The model under review builds one solid part; all positions refer to its coordinate system, in mm. Round coordinates to 2 decimals unless told otherwise and drop trailing zeros. Order: outer loops, then holes, each group sorted by start corner. A loop starts at its lowest first (then second) coordinate and runs counter-clockwise, first axis right, second up.
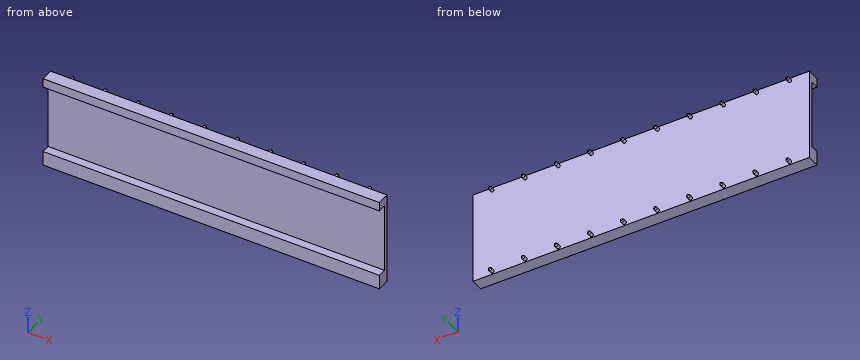
from build123d import *
from OCP.BRepFilletAPI import BRepFilletAPI_MakeChamfer

# Parameters (mm, degrees)
SKETCH1_W                   = 488.315
SKETCH1_H                   = 133.985
BOSS_EXTRUDE1_DEPTH         = 6.0452
SKETCH2_R                   = 2.4765
BOSS_EXTRUDE2_DEPTH         = 7.62
CHAMFER1_SIZE               = 2.032
CHAMFER1_SIZE2              = 1.173175747
LPATTERN1_COUNT             = 5
LPATTERN1_PITCH             = 95.9866
CHAMFER1_OF_LPATTERN1_SIZE  = 2.032
CHAMFER1_OF_LPATTERN1_SIZE2 = 1.173175747
SKETCH3_W                   = 20.955
SKETCH3_H                   = 12.065
SKETCH3_W_2                 = 13.0048
BOSS_EXTRUDE3_DEPTH         = 488.315


with BuildPart() as part:
    # Sketch1 → Boss-Extrude1 (new body)
    with BuildSketch(Plane(origin=(0, 0, 0), x_dir=(1, 0, 0), z_dir=(0, 1, 0))):
        with Locations((244.1575, -66.9925)):
            Rectangle(SKETCH1_W, SKETCH1_H)
    extrude(amount=-BOSS_EXTRUDE1_DEPTH)

    # Sketch2 → Boss-Extrude2 (add)
    with BuildSketch(Plane(origin=(0, 0, 0), x_dir=(1, 0, 0), z_dir=(0, 1, 0))):
        with Locations(Location((28.1305, -4.0005, 0), (0, 0, 90))):
            Circle(SKETCH2_R)
        with Locations(Location((76.1365, -4.0005, 0), (0, 0, 90))):
            Circle(SKETCH2_R)
        with Locations(Location((28.1305, -129.9845, 0), (0, 0, 90))):
            Circle(SKETCH2_R)
        with Locations(Location((76.1365, -129.9845, 0), (0, 0, 90))):
            Circle(SKETCH2_R)
    boss_extrude2 = extrude(amount=BOSS_EXTRUDE2_DEPTH)

    # Chamfer1: one chamfer whose edges measure the first distance from different faces: ONE call of the kernel's chamfer builder (chamfer() names one face for all edges)
    chamfer1_edges_1 = [part.edges().sort_by_distance(p)[0] for p in [
        (28.1305, 7.62, 6.477),
    ]]
    chamfer1_side_1 = [part.faces().sort_by_distance(p)[0] for p in [
        (28.1305, 3.81, 6.477),
    ]]
    chamfer1_edges_2 = [part.edges().sort_by_distance(p)[0] for p in [
        (76.1365, 7.62, 6.477),
    ]]
    chamfer1_side_2 = [part.faces().sort_by_distance(p)[0] for p in [
        (76.1365, 3.81, 6.477),
    ]]
    chamfer1_edges_3 = [part.edges().sort_by_distance(p)[0] for p in [
        (28.1305, 7.62, 132.461),
    ]]
    chamfer1_side_3 = [part.faces().sort_by_distance(p)[0] for p in [
        (28.1305, 3.81, 132.461),
    ]]
    chamfer1_edges_4 = [part.edges().sort_by_distance(p)[0] for p in [
        (76.1365, 7.62, 132.461),
    ]]
    chamfer1_side_4 = [part.faces().sort_by_distance(p)[0] for p in [
        (76.1365, 3.81, 132.461),
    ]]
    chamfer1 = BRepFilletAPI_MakeChamfer(part.part.solid().wrapped)
    for e in chamfer1_edges_1:
        chamfer1.Add(CHAMFER1_SIZE, CHAMFER1_SIZE2, e.wrapped, chamfer1_side_1[0].wrapped)  # the first distance lies on this face
    for e in chamfer1_edges_2:
        chamfer1.Add(CHAMFER1_SIZE, CHAMFER1_SIZE2, e.wrapped, chamfer1_side_2[0].wrapped)  # the first distance lies on this face
    for e in chamfer1_edges_3:
        chamfer1.Add(CHAMFER1_SIZE, CHAMFER1_SIZE2, e.wrapped, chamfer1_side_3[0].wrapped)  # the first distance lies on this face
    for e in chamfer1_edges_4:
        chamfer1.Add(CHAMFER1_SIZE, CHAMFER1_SIZE2, e.wrapped, chamfer1_side_4[0].wrapped)  # the first distance lies on this face
    add(Compound.cast(chamfer1.Shape()), mode=Mode.REPLACE)

    # LPattern1: Boss-Extrude2 ×5
    with Locations(*[(i * LPATTERN1_PITCH, 0, 0) for i in range(1, LPATTERN1_COUNT)]):
        add(boss_extrude2)

    # Chamfer1 of LPattern1: one chamfer whose edges measure the first distance from different faces: ONE call of the kernel's chamfer builder (chamfer() names one face for all edges)
    chamfer1_of_lpattern1_edges_1 = [part.edges().sort_by_distance(p)[0] for p in [
        (124.1171, 7.62, 6.477),
    ]]
    chamfer1_of_lpattern1_side_1 = [part.faces().sort_by_distance(p)[0] for p in [
        (124.1171, 3.81, 6.477),
    ]]
    chamfer1_of_lpattern1_edges_2 = [part.edges().sort_by_distance(p)[0] for p in [
        (172.1231, 7.62, 6.477),
    ]]
    chamfer1_of_lpattern1_side_2 = [part.faces().sort_by_distance(p)[0] for p in [
        (172.1231, 3.81, 6.477),
    ]]
    chamfer1_of_lpattern1_edges_3 = [part.edges().sort_by_distance(p)[0] for p in [
        (124.1171, 7.62, 132.461),
    ]]
    chamfer1_of_lpattern1_side_3 = [part.faces().sort_by_distance(p)[0] for p in [
        (124.1171, 3.81, 132.461),
    ]]
    chamfer1_of_lpattern1_edges_4 = [part.edges().sort_by_distance(p)[0] for p in [
        (172.1231, 7.62, 132.461),
    ]]
    chamfer1_of_lpattern1_side_4 = [part.faces().sort_by_distance(p)[0] for p in [
        (172.1231, 3.81, 132.461),
    ]]
    chamfer1_of_lpattern1_edges_5 = [part.edges().sort_by_distance(p)[0] for p in [
        (220.1037, 7.62, 6.477),
    ]]
    chamfer1_of_lpattern1_side_5 = [part.faces().sort_by_distance(p)[0] for p in [
        (220.1037, 3.81, 6.477),
    ]]
    chamfer1_of_lpattern1_edges_6 = [part.edges().sort_by_distance(p)[0] for p in [
        (268.1097, 7.62, 6.477),
    ]]
    chamfer1_of_lpattern1_side_6 = [part.faces().sort_by_distance(p)[0] for p in [
        (268.1097, 3.81, 6.477),
    ]]
    chamfer1_of_lpattern1_edges_7 = [part.edges().sort_by_distance(p)[0] for p in [
        (220.1037, 7.62, 132.461),
    ]]
    chamfer1_of_lpattern1_side_7 = [part.faces().sort_by_distance(p)[0] for p in [
        (220.1037, 3.81, 132.461),
    ]]
    chamfer1_of_lpattern1_edges_8 = [part.edges().sort_by_distance(p)[0] for p in [
        (268.1097, 7.62, 132.461),
    ]]
    chamfer1_of_lpattern1_side_8 = [part.faces().sort_by_distance(p)[0] for p in [
        (268.1097, 3.81, 132.461),
    ]]
    chamfer1_of_lpattern1_edges_9 = [part.edges().sort_by_distance(p)[0] for p in [
        (316.0903, 7.62, 6.477),
    ]]
    chamfer1_of_lpattern1_side_9 = [part.faces().sort_by_distance(p)[0] for p in [
        (316.0903, 3.81, 6.477),
    ]]
    chamfer1_of_lpattern1_edges_10 = [part.edges().sort_by_distance(p)[0] for p in [
        (364.0963, 7.62, 6.477),
    ]]
    chamfer1_of_lpattern1_side_10 = [part.faces().sort_by_distance(p)[0] for p in [
        (364.0963, 3.81, 6.477),
    ]]
    chamfer1_of_lpattern1_edges_11 = [part.edges().sort_by_distance(p)[0] for p in [
        (316.0903, 7.62, 132.461),
    ]]
    chamfer1_of_lpattern1_side_11 = [part.faces().sort_by_distance(p)[0] for p in [
        (316.0903, 3.81, 132.461),
    ]]
    chamfer1_of_lpattern1_edges_12 = [part.edges().sort_by_distance(p)[0] for p in [
        (364.0963, 7.62, 132.461),
    ]]
    chamfer1_of_lpattern1_side_12 = [part.faces().sort_by_distance(p)[0] for p in [
        (364.0963, 3.81, 132.461),
    ]]
    chamfer1_of_lpattern1_edges_13 = [part.edges().sort_by_distance(p)[0] for p in [
        (412.0769, 7.62, 6.477),
    ]]
    chamfer1_of_lpattern1_side_13 = [part.faces().sort_by_distance(p)[0] for p in [
        (412.0769, 3.81, 6.477),
    ]]
    chamfer1_of_lpattern1_edges_14 = [part.edges().sort_by_distance(p)[0] for p in [
        (460.0829, 7.62, 6.477),
    ]]
    chamfer1_of_lpattern1_side_14 = [part.faces().sort_by_distance(p)[0] for p in [
        (460.0829, 3.81, 6.477),
    ]]
    chamfer1_of_lpattern1_edges_15 = [part.edges().sort_by_distance(p)[0] for p in [
        (412.0769, 7.62, 132.461),
    ]]
    chamfer1_of_lpattern1_side_15 = [part.faces().sort_by_distance(p)[0] for p in [
        (412.0769, 3.81, 132.461),
    ]]
    chamfer1_of_lpattern1_edges_16 = [part.edges().sort_by_distance(p)[0] for p in [
        (460.0829, 7.62, 132.461),
    ]]
    chamfer1_of_lpattern1_side_16 = [part.faces().sort_by_distance(p)[0] for p in [
        (460.0829, 3.81, 132.461),
    ]]
    chamfer1_of_lpattern1 = BRepFilletAPI_MakeChamfer(part.part.solid().wrapped)
    for e in chamfer1_of_lpattern1_edges_1:
        chamfer1_of_lpattern1.Add(CHAMFER1_OF_LPATTERN1_SIZE, CHAMFER1_OF_LPATTERN1_SIZE2, e.wrapped, chamfer1_of_lpattern1_side_1[0].wrapped)  # the first distance lies on this face
    for e in chamfer1_of_lpattern1_edges_2:
        chamfer1_of_lpattern1.Add(CHAMFER1_OF_LPATTERN1_SIZE, CHAMFER1_OF_LPATTERN1_SIZE2, e.wrapped, chamfer1_of_lpattern1_side_2[0].wrapped)  # the first distance lies on this face
    for e in chamfer1_of_lpattern1_edges_3:
        chamfer1_of_lpattern1.Add(CHAMFER1_OF_LPATTERN1_SIZE, CHAMFER1_OF_LPATTERN1_SIZE2, e.wrapped, chamfer1_of_lpattern1_side_3[0].wrapped)  # the first distance lies on this face
    for e in chamfer1_of_lpattern1_edges_4:
        chamfer1_of_lpattern1.Add(CHAMFER1_OF_LPATTERN1_SIZE, CHAMFER1_OF_LPATTERN1_SIZE2, e.wrapped, chamfer1_of_lpattern1_side_4[0].wrapped)  # the first distance lies on this face
    for e in chamfer1_of_lpattern1_edges_5:
        chamfer1_of_lpattern1.Add(CHAMFER1_OF_LPATTERN1_SIZE, CHAMFER1_OF_LPATTERN1_SIZE2, e.wrapped, chamfer1_of_lpattern1_side_5[0].wrapped)  # the first distance lies on this face
    for e in chamfer1_of_lpattern1_edges_6:
        chamfer1_of_lpattern1.Add(CHAMFER1_OF_LPATTERN1_SIZE, CHAMFER1_OF_LPATTERN1_SIZE2, e.wrapped, chamfer1_of_lpattern1_side_6[0].wrapped)  # the first distance lies on this face
    for e in chamfer1_of_lpattern1_edges_7:
        chamfer1_of_lpattern1.Add(CHAMFER1_OF_LPATTERN1_SIZE, CHAMFER1_OF_LPATTERN1_SIZE2, e.wrapped, chamfer1_of_lpattern1_side_7[0].wrapped)  # the first distance lies on this face
    for e in chamfer1_of_lpattern1_edges_8:
        chamfer1_of_lpattern1.Add(CHAMFER1_OF_LPATTERN1_SIZE, CHAMFER1_OF_LPATTERN1_SIZE2, e.wrapped, chamfer1_of_lpattern1_side_8[0].wrapped)  # the first distance lies on this face
    for e in chamfer1_of_lpattern1_edges_9:
        chamfer1_of_lpattern1.Add(CHAMFER1_OF_LPATTERN1_SIZE, CHAMFER1_OF_LPATTERN1_SIZE2, e.wrapped, chamfer1_of_lpattern1_side_9[0].wrapped)  # the first distance lies on this face
    for e in chamfer1_of_lpattern1_edges_10:
        chamfer1_of_lpattern1.Add(CHAMFER1_OF_LPATTERN1_SIZE, CHAMFER1_OF_LPATTERN1_SIZE2, e.wrapped, chamfer1_of_lpattern1_side_10[0].wrapped)  # the first distance lies on this face
    for e in chamfer1_of_lpattern1_edges_11:
        chamfer1_of_lpattern1.Add(CHAMFER1_OF_LPATTERN1_SIZE, CHAMFER1_OF_LPATTERN1_SIZE2, e.wrapped, chamfer1_of_lpattern1_side_11[0].wrapped)  # the first distance lies on this face
    for e in chamfer1_of_lpattern1_edges_12:
        chamfer1_of_lpattern1.Add(CHAMFER1_OF_LPATTERN1_SIZE, CHAMFER1_OF_LPATTERN1_SIZE2, e.wrapped, chamfer1_of_lpattern1_side_12[0].wrapped)  # the first distance lies on this face
    for e in chamfer1_of_lpattern1_edges_13:
        chamfer1_of_lpattern1.Add(CHAMFER1_OF_LPATTERN1_SIZE, CHAMFER1_OF_LPATTERN1_SIZE2, e.wrapped, chamfer1_of_lpattern1_side_13[0].wrapped)  # the first distance lies on this face
    for e in chamfer1_of_lpattern1_edges_14:
        chamfer1_of_lpattern1.Add(CHAMFER1_OF_LPATTERN1_SIZE, CHAMFER1_OF_LPATTERN1_SIZE2, e.wrapped, chamfer1_of_lpattern1_side_14[0].wrapped)  # the first distance lies on this face
    for e in chamfer1_of_lpattern1_edges_15:
        chamfer1_of_lpattern1.Add(CHAMFER1_OF_LPATTERN1_SIZE, CHAMFER1_OF_LPATTERN1_SIZE2, e.wrapped, chamfer1_of_lpattern1_side_15[0].wrapped)  # the first distance lies on this face
    for e in chamfer1_of_lpattern1_edges_16:
        chamfer1_of_lpattern1.Add(CHAMFER1_OF_LPATTERN1_SIZE, CHAMFER1_OF_LPATTERN1_SIZE2, e.wrapped, chamfer1_of_lpattern1_side_16[0].wrapped)  # the first distance lies on this face
    add(Compound.cast(chamfer1_of_lpattern1.Shape()), mode=Mode.REPLACE)

    # Sketch3 → Boss-Extrude3 (add)
    with BuildSketch(Plane(origin=(0, 0, 0), x_dir=(0, 0, -1), z_dir=(1, 0, 0))):
        with Locations((-10.4775, -12.0777)):
            Rectangle(SKETCH3_W, SKETCH3_H)
        with Locations((-127.4826, -12.0777)):
            Rectangle(SKETCH3_W_2, SKETCH3_H)
    extrude(amount=BOSS_EXTRUDE3_DEPTH)


solid = part.part
(1) Clearance check with flat-ended pins moving along their axes: P1, Ø6, axis at x = 276, y = -1.5, coming from the -Z side; P2, Ø4, axis at x = 135.5, z = 101.5, coming from the +Y side; P3, Ø12, axis at x = 243.5, z = 69.5, coming from the -Y side; P4, Ø5, axis at x = 292, y = 4, coming from the +Z side. State where each tip first meets the part, or that it passes through.
(2) We need section B-B (z = 114.5). Give the boundary of the cut face in (x, y) (3 decimals), and give its area (3 significant figures).
(3) To check wall thickness, follow L1, parallel to Z at x = 43, y = -6.25 (3 decimals); L2, parallel to Y at x = 249.5, z = 92.5; L3, parallel to Y at x = 22.5, z = 20. State the ranges of each line that lie inside material, in increasing order.
(4) We need section A-A (x = 201.5). Give the boundary of the cut face in (y, z) (3 decimals).
Verdict:
1. P1: stops at z = 0
1. P2: stops at y = 0
1. P3: stops at y = -6.05
1. P4: passes through
2. outline: (0, -6.045) - (488.315, -6.045) - (488.315, 0) - (0, 0) - close
2. area: 2,950 mm2
3. L1: z = 0 to 20.955, 120.98 to 133.985
3. L2: y = -6.05 to 0
3. L3: y = -18.11 to 0
4. outline: (-18.11, 0) - (0, 0) - (0, 133.985) - (-18.11, 133.985) - (-18.11, 120.98) - (-6.045, 120.98) - (-6.045, 20.955) - (-18.11, 20.955) - close
